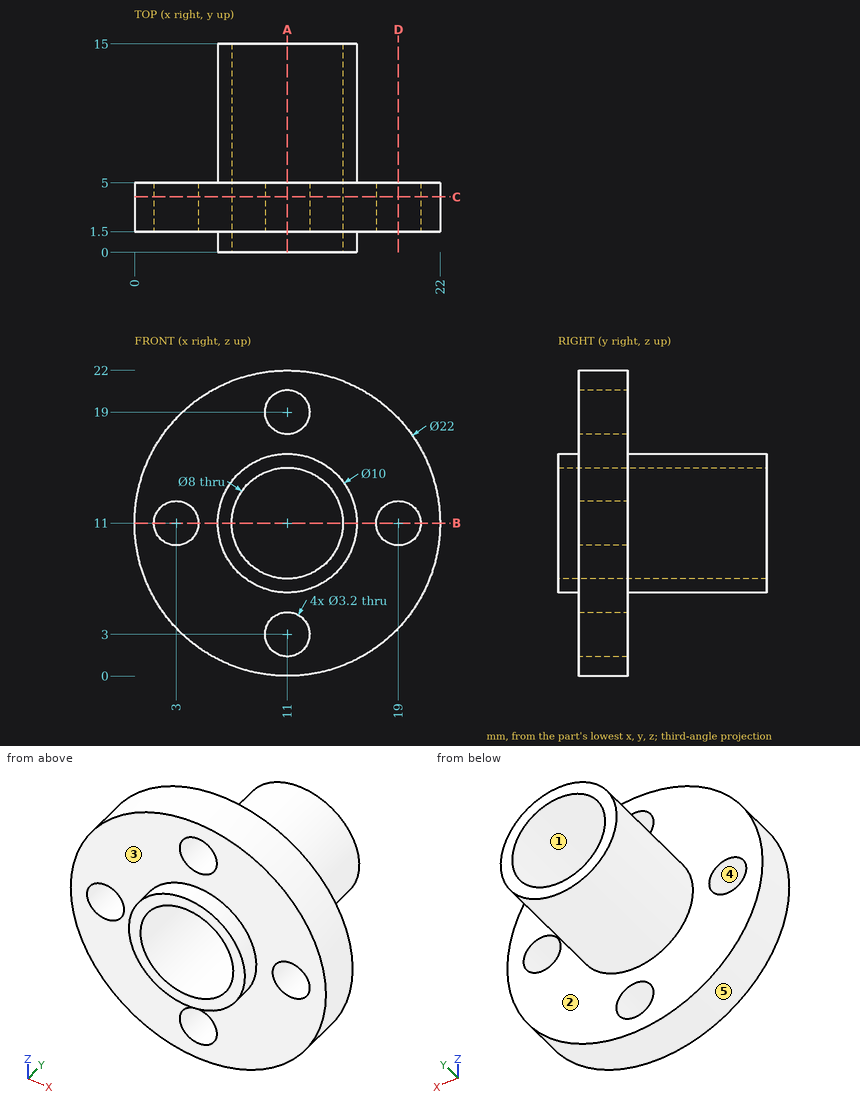
Verification items for this drawing (mm, ordinates from the low corner). A direction names the side the tool comes from. Coordinates: 2 decimals unless noted, no trailing zeros. Order: outer loops, then holes, each group sorted by start corner. A loop starts at its lowest first (then second) coordinate and runs counter-clockwise, first axis right, second up.
Q1. Draft check along Z on the marked faces 3, 4 and 5. Enter one of: released by +Z, released by -Z, zero draft, split by the parting line, or undercut.
Reply:
face 3: zero draft
face 4: undercut
face 5: split by the parting line
Q2. Sectioned sample at B-B on z = 11. Record the cut outline in (x, y), and give its area (3 significant figures).
Reply:
outline: (0, 1.5) - (1.4, 1.5) - (1.4, 5) - (0, 5) - close; (4.6, 1.5) - (6, 1.5) - (6, 0) - (7, 0) - (7, 15) - (6, 15) - (6, 5) - (4.6, 5) - close; (15, 0) - (16, 0) - (16, 1.5) - (17.4, 1.5) - (17.4, 5) - (16, 5) - (16, 15) - (15, 15) - close; (20.6, 1.5) - (22, 1.5) - (22, 5) - (20.6, 5) - close
area: 49.6 mm2
Q3. Tool access check on the marked faces 1 and 2. Record the directions out of +Z, -Z, +X, -X, +Y, -Y that give a thin tool (end or side, any length) a straight path to the whole face; none if there is none.
Reply:
face 1: +Y, -Y
face 2: +Y
Q4. Depth check by flat-ended pin: pin 1 Ø2.5 at (x, z) = (11, 3) entering from -Y; pin 2 Ø2 at (y, z) = (1.5, 15.5) entering from +X; pin 3 Ø2 at (y, z) = (12.5, 9) entering from +X; pin 4 Ø5 at (x, y) = (16, 12.5) entering from -Z. Enter the tip coordinate at first touch or a pass-through.
Reply:
pin 1: passes through
pin 2: stops at x = 21.43
pin 3: stops at x = 15.9
pin 4: stops at z = 6.67
Q5. Sectioned sample at C-C on y = 4. Record the cut outline in (x, z), and give its area (3 significant figures).
Reply:
outline: circle Ø22 at (11, 11); hole circle Ø3.2 at (3, 11); hole circle Ø8 at (11, 11); hole circle Ø3.2 at (11, 3); hole circle Ø3.2 at (11, 19); hole circle Ø3.2 at (19, 11)
area: 298 mm2
Q6. Sectioned sample at D-D on x = 19. Record the cut outline in (y, z), and give its area (3 significant figures).
Reply:
outline: (1.5, 3.45) - (5, 3.45) - (5, 9.4) - (1.5, 9.4) - close; (1.5, 12.6) - (5, 12.6) - (5, 18.55) - (1.5, 18.55) - close
area: 41.6 mm2
Q7. Sectioned sample at A-A on x = 11. Record the cut outline in (y, z), and give its area (3 significant figures).
Reply:
outline: (0, 6) - (1.5, 6) - (1.5, 4.6) - (5, 4.6) - (5, 6) - (15, 6) - (15, 7) - (0, 7) - close; (0, 15) - (15, 15) - (15, 16) - (5, 16) - (5, 17.4) - (1.5, 17.4) - (1.5, 16) - (0, 16) - close; (1.5, 0) - (5, 0) - (5, 1.4) - (1.5, 1.4) - close; (1.5, 20.6) - (5, 20.6) - (5, 22) - (1.5, 22) - close
area: 49.6 mm2
Q8. Thickness scan on probe 1 along X at (y, z) = (3.45, 11); probe 2 along X at (y, z) = (7.75, 11); probe 3 along Y at (x, z) = (14, 3). Record the ranges inside material, lowest first.
Reply:
probe 1: x = 0 to 1.4, 4.6 to 7, 15 to 17.4, 20.6 to 22
probe 2: x = 6 to 7, 15 to 16
probe 3: y = 1.5 to 5
